```python
from build123d import *

# Parameters (mm, degrees)
SKETCH1_W             = 31.7
SKETCH1_H             = 31.7
BOSS_EXTRUDE1_DEPTH   = 3
SKETCH2_R             = 14.5
BOSS_EXTRUDE2_DEPTH   = 61
F_3_0MM_DOWEL_HOLE1_D = 3
SKETCH6_R             = 3
CUT_EXTRUDE1_DEPTH    = 65


with BuildPart() as part:
    # Sketch1 → Boss-Extrude1 (new body)
    with BuildSketch(Plane(origin=(0, 0, 0), x_dir=(1, 0, 0), z_dir=(0, 1, 0))):
        Rectangle(SKETCH1_W, SKETCH1_H)
    extrude(amount=BOSS_EXTRUDE1_DEPTH)

    # Sketch2 → Boss-Extrude2 (add)
    with BuildSketch(Plane(origin=(0, 3, 0), x_dir=(1, 0, 0), z_dir=(0, 1, 0))):
        Circle(SKETCH2_R)
    extrude(amount=BOSS_EXTRUDE2_DEPTH)

    # Ø3.0mm Dowel Hole1 (through all)
    with Locations(Plane(origin=(0, 0, 0), x_dir=(-1, 0, 0), z_dir=(0, -1, 0))):
        with Locations((12.551145366, -12.551145366), (-12.551145366, -12.551145366), (12.551145366, 12.551145366), (-12.551145366, 12.551145366)):
            Hole(F_3_0MM_DOWEL_HOLE1_D / 2)

    # Sketch6 → Cut-Extrude1 (cut, through all)
    with BuildSketch(Plane(origin=(0, 64, 0), x_dir=(1, 0, 0), z_dir=(0, 1, 0))):
        Circle(SKETCH6_R)
    extrude(amount=-CUT_EXTRUDE1_DEPTH, mode=Mode.SUBTRACT)


solid = part.part
```
Geometry: final body of the model. Coordinates: model frame, mm. A direction names the side the tool comes from. Round coordinates to 2 decimals unless told otherwise and drop trailing zeros. Order: outer loops, then holes, each group sorted by start corner. A loop starts at its lowest first (then second) coordinate and runs counter-clockwise, first axis right, second up. Notation, with made-up numbers: (-28.75, 24.25) - (3.25, 24.25) arc R19 ccw to (3.25, 51.25) - close; hole circle Ø9 at (47.5, -32.75). An arc over 180 degrees is marked (long way). Use CSV: the item, a comma, the result in double quotes. Start each with the question number.
Q1. Material intervals for line 1 along X through (y, z) = (41, 0); line 2 along X through (y, z) = (49.5, 1.5), sorted ascending. Write a range as from..to.
Q2. Section query B-B (z = 0). Return loops of the section in (x, y), and give its area (3 significant figures).
Q3. Access query for faces 5 (the face through (-7, 3, -13)), 6 (the face through (-0.2, 64, -3.4)). Directions: +Z, -Z, +X, -X, +Y, -Y. A direction counts if a zero-diameter tool reaches every point of the face in a straight line with its end or side. Return the directions, or none.
Q4. Section query D-D (x = -8.5). Return loops of the section in (y, z).
Q5. Mould query, pull axis Z, two halves, no side actions, for faces 1 (the face through (6.691, 33.073, 12.864)), 2 (the face through (-15.85, 1, 0)), 3 (the face through (0, 1, -15.85)), 4 (the face through (-14.05, 1.52, 12.49)). Classes: +Z half, -Z half, draft (parallel to the pull), parting line (faces both ways), or undercut.
Q6. Section query A-A (x = 0). Return loops of the section in (y, z), and give its area (3 significant figures).
Q7. Section query C-C (y = 42.5). Return loops of the section in (x, z), and give its area (3 significant figures).
Q8. First-contact query: pin 1 (3 mm diameter, centred on x = -11.5, y = 16.5, fed in from +Z); pin 2 (4 mm diameter, centred on x = -10, y = 15, fed in from +Z); pin 3 (4 mm diameter, centred on x = 6.5, y = 35.5, fed in from +Z); pin 4 (2.5 mm diameter, centred on x = -12.55, z = -12.55, fed in from -Y). Flat tips, straight axial feed; report the tip coordinate or a pass-through.
Result set:
1,line 1,"x = -14.5..-3, 3..14.5"
1,line 2,"x = -14.42..-2.6, 2.6..14.42"
2,outline,"(-15.85, 0) - (-3, 0) - (-3, 64) - (-14.5, 64) - (-14.5, 3) - (-15.85, 3) - close; (3, 0) - (15.85, 0) - (15.85, 3) - (14.5, 3) - (14.5, 64) - (3, 64) - close"
2,area,"1,480 mm2"
3,face 5,"+Y"
3,face 6,"+Z, -Z, +X, -X, +Y"
4,outline,"(0, -15.85) - (3, -15.85) - (3, -11.75) - (64, -11.75) - (64, 11.75) - (3, 11.75) - (3, 15.85) - (0, 15.85) - close"
5,face 1,"parting line"
5,face 2,"draft"
5,face 3,"-Z half"
5,face 4,"undercut"
6,outline,"(0, -15.85) - (3, -15.85) - (3, -14.5) - (64, -14.5) - (64, -3) - (0, -3) - close; (0, 3) - (64, 3) - (64, 14.5) - (3, 14.5) - (3, 15.85) - (0, 15.85) - close"
6,area,"1,480 mm2"
7,outline,"circle Ø29 at (0, 0); hole circle Ø6 at (0, 0)"
7,area,"632 mm2"
8,pin 1,"stops at z = 10.5"
8,pin 2,"stops at z = 12.09"
8,pin 3,"stops at z = 13.78"
8,pin 4,"passes through"
